Geometry check sheet. Reference: the model listing, model coordinates, mm. Give positions to 0.01 mm unless a question says otherwise; leave off trailing zeros. Loops run counter-clockwise (first coordinate to the right, second up) from the corner with the lowest first, then second, coordinate; pieces in that order, holes last. Notation, with made-up numbers: (-20, 68.5) - (18, 68.5) arc R16 ccw to (18, 74.5) - close; hole circle Ø9 at (-24, 78). An arc over 180 degrees is marked (long way). Use a Markdown table: item, result. Add a question column.
1. Cross-section at D-D on x = -9. Enter the section's corners in (y, z).
2. Cross-section at B-B on y = -9.5. Enter the section's corners in (x, z), and give its area (3 significant figures).
3. Cross-section at C-C on y = 6.5. Enter the section's corners in (x, z).
4. Material ranges on L1, parallel to Y at x = 10.5, z = -0.6; L2, parallel to X at y = 0, z = -0.4; L3, parallel to X at y = -4, z = -0.2, recorded low to high.
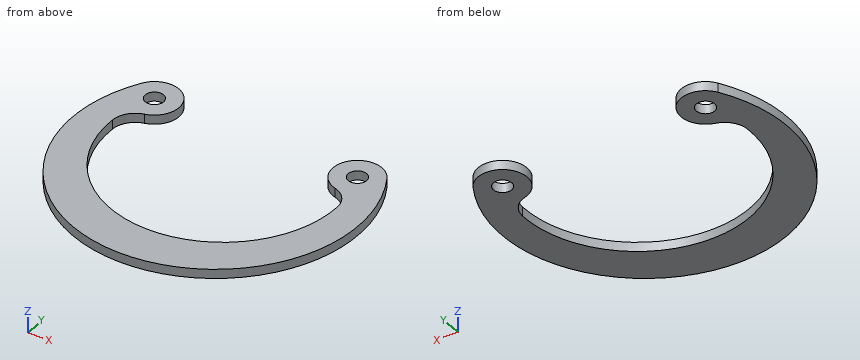
from build123d import *

# Parameters (mm, degrees)
SKETCH_1_R      = 1
EXTRUDE_1_DEPTH = 1


with BuildPart() as part:
    # Эскиз1 → Бобышка-Вытянуть1 (new body)
    with BuildSketch(Plane.XY):
        with BuildLine():
            ThreePointArc((-13.365556031, 7.849325575), (0, -15.5), (13.365556031, 7.849325575))
            ThreePointArc((13.365556031, 7.849325575), (8.94560833, 8.110945689), (10.386242309, 3.924186023))
            ThreePointArc((10.386242309, 3.924186023), (11.7073461, 3.058360422), (12.245730412, 1.573398627))
            ThreePointArc((12.245730412, 1.573398627), (0, -11), (-12.245730412, 1.573398627))
            ThreePointArc((-12.245730412, 1.573398627), (-11.7073461, 3.058360422), (-10.386242309, 3.924186023))
            ThreePointArc((-10.386242309, 3.924186023), (-8.94560833, 8.110945689), (-13.365556031, 7.849325575))
        make_face()
        with Locations((-11.067971811, 6.5)):
            Circle(SKETCH_1_R, mode=Mode.SUBTRACT)
        with Locations((11.067971811, 6.5)):
            Circle(SKETCH_1_R, mode=Mode.SUBTRACT)
    extrude(amount=-EXTRUDE_1_DEPTH)


solid = part.part
Values found:
| question | item | result |
|---|---|---|
| 1 | outline | (-12.62, -1) - (-7.06, -1) - (-7.06, 0) - (-12.62, 0) - close; (4.82, -1) - (8.18, -1) - (8.18, 0) - (4.82, 0) - close |
| 2 | outline | (-12.25, -1) - (-5.87, -1) - (-5.87, 0) - (-12.25, 0) - close; (5.87, -1) - (12.25, -1) - (12.25, 0) - (5.87, 0) - close |
| 2 | area | 12.7 mm2 |
| 3 | outline | (-14.07, -1) - (-12.07, -1) - (-12.07, 0) - (-14.07, 0) - close; (-10.07, -1) - (-8.4, -1) - (-8.4, 0) - (-10.07, 0) - close; (8.4, -1) - (10.07, -1) - (10.07, 0) - (8.4, 0) - close; (12.07, -1) - (14.07, -1) - (14.07, 0) - (12.07, 0) - close |
| 4 | L1 | y = -11.4 to -5.06, 3.89 to 5.68, 7.32 to 9.1 |
| 4 | L2 | x = -15.5 to -12.19, 12.19 to 15.5 |
| 4 | L3 | x = -14.97 to -11.07, 11.07 to 14.97 |
